```python
from build123d import *

# Parameters (mm, degrees)
SKETCH_1_R           = 2
EXTRUDE_1_DEPTH      = 3
SKETCH_2_R           = 2
EXTRUDE_2_DEPTH      = 3
EXTRUDE_3_DEPTH      = 5
EXTRUDE_3_DEPTH_BACK = 5
SKETCH_4_R           = 2
CUT_EXTRUDE_1_DEPTH  = 31.046838436


with BuildPart() as part:
    # Sketch 1 → Extrude 1 (new body)
    with BuildSketch(Plane(origin=(0, 0, 0), x_dir=(1, 0, 0), z_dir=(0, 1, 0))):
        with BuildLine():
            Line((-11.75, 5.5), (11.75, 5.5))
            ThreePointArc((11.75, 5.5), (16.808303364, 2.159529364), (15.72220169, -3.804157427))
            Line((15.72220169, -3.804157427), (5, -15))
            Line((5, -15), (-5, -15))
            Line((-5, -15), (-15.72220169, -3.804157427))
            ThreePointArc((-15.72220169, -3.804157427), (-16.808303364, 2.159529364), (-11.75, 5.5))
        make_face()
        with Locations(Location((-11.75, 0, 0), (0, 0, 270))):
            Circle(SKETCH_1_R, mode=Mode.SUBTRACT)
        with Locations(Location((11.75, 0, 0), (0, 0, 270))):
            Circle(SKETCH_1_R, mode=Mode.SUBTRACT)
    extrude(amount=EXTRUDE_1_DEPTH)

    # Sketch 2 → Extrude 2 (add)
    with BuildSketch(Plane.XY.offset(15)):
        with BuildLine():
            Line((11.75, 22.5), (-11.75, 22.5))
            ThreePointArc((-11.75, 22.5), (-16.717422464, 19.361083239), (-16.014908335, 13.527168749))
            Line((-16.014908335, 13.527168749), (-5, 0))
            Line((-5, 0), (5, 0))
            Line((5, 0), (16.014908335, 13.527168749))
            ThreePointArc((16.014908335, 13.527168749), (16.717422464, 19.361083239), (11.75, 22.5))
        make_face()
        with Locations((11.75, 17)):
            Circle(SKETCH_2_R, mode=Mode.SUBTRACT)
        with Locations((-11.75, 17)):
            Circle(SKETCH_2_R, mode=Mode.SUBTRACT)
    extrude(amount=-EXTRUDE_2_DEPTH)

    # Sketch 3 → Extrude 3 (add, two sides: drawn at the far end of the back side and taken through both)
    with BuildSketch(Plane(origin=(0, 0, 0), x_dir=(0, 0, -1), z_dir=(1, 0, 0)).offset(-EXTRUDE_3_DEPTH_BACK)):
        Polygon((-12, 13.527168749), (-3.804157427, 3), (-12, 3), align=None)
    extrude(amount=EXTRUDE_3_DEPTH + EXTRUDE_3_DEPTH_BACK)

    # Sketch 4 → Cut-Extrude 1 (cut, through all)
    with BuildSketch(Plane(origin=(0, 3, 0), x_dir=(1, 0, 0), z_dir=(0, 1, 0))):
        with Locations(Location((0, -7.947430558, 0), (0, 0, 90))):
            Circle(SKETCH_4_R)
    extrude(amount=CUT_EXTRUDE_1_DEPTH, mode=Mode.SUBTRACT)


solid = part.part
```
Could you check a few things on this model? Use its own coordinates, in mm. A direction names the side the tool comes from. Round coordinates to 2 decimals unless told otherwise and drop trailing zeros. Write each loop counter-clockwise with the first axis right and the second up, starting at its lowest first coordinate (ties: lowest second). Pieces come first, ordered by that corner, then holes. Notation, with made-up numbers: M 35.25,70.5 L 92.25,70.5 A21 ccw 92.25,100.5 Z; hole C 51.25,74 d3. An arc over 180 degrees is marked long. Answer in a Markdown table with one row per item. Add a question column.
Q1. If I drill on line 1 (X direction, y = 2.25, z = 0); line 2 (Z direction, x = 11, y = 8); line 3 (Y direction, x = 11, z = 7.5), over which ranges is the centre line in solid material (lowest first)? Write a range as from..to.
Q2. Imagine slicing it at D-D (x = -10.5). Please give me the cut outline in (y, z), then the cut area to 3 significant figures.
Q3. If we mould it in two halves opening along Y, with no side actions, what happens to faces 1 (the cylindrical face through (-16.84, 1.48, -2.08)), 2 (the flat face through (0, 3, 8)), 3 (the cylindrical face through (11.49, 18.983, 13.521)), 4 (the cylindrical face through (16.754, 19.282, 13.521))? For each: +Y half, -Y half, draft (parallel to the pull), parting line (faces both ways), or undercut.
Q4. Will these pins go through, and if not, where does the flat tip stop? pin 1 Ø5 at (x, y) = (-11.75, 17) entering from -Z; pin 2 Ø2.5 at (x, z) = (11.75, 0) entering from -Y; pin 3 Ø2 at (x, z) = (0, 8.5) entering from +Y; pin 4 Ø9 at (y, z) = (6.5, 10) entering from -X.
Q5. On a 3-axis mill with a long thin cutter (end or side, diameter ignored), from which of +Z, -Z, +X, -X, +Y, -Y can I reach the whole of each face in a straight line? I mean faces 5 (the flat face through (0, 15, 12)), 6 (the flat face through (10.44, 1.48, 9.32)), 7 (the flat face through (5, 6, 10)). Say none if no direction works.
Q6. Imagine slicing it at B-B (z = 0.75). Please give me the cut outline in (x, y), then the cut area to 3 significant figures.
Q7. Imagine slicing it at C-C (y = 4.75). Please give me the cut outline in (x, z), then the cut area to 3 significant figures.
Q8. Imagine slicing it at A-A (x = 3). Please give me the cut outline in (y, z), then the cut area to 3 significant figures.
Values:
| question | item | result |
|---|---|---|
| 1 | line 1 | -17.25..-13.75, -9.75..9.75, 13.75..17.25 |
| 1 | line 2 | 12..15 |
| 1 | line 3 | 0..3 |
| 2 | outline | M 0,-5.5 L 3,-5.5 L 3,-1.56 L 0,-1.56 Z; M 0,1.56 L 3,1.56 L 3,9.26 L 0,9.26 Z; M 6.75,12 L 15.44,12 L 15.44,15 L 6.75,15 Z; M 18.56,12 L 22.5,12 L 22.5,15 L 18.56,15 Z |
| 2 | area | 72.8 mm^2 |
| 3 | face 1 | draft |
| 3 | face 2 | +Y half |
| 3 | face 3 | undercut |
| 3 | face 4 | parting line |
| 4 | pin 1 | z = 12 |
| 4 | pin 2 | through |
| 4 | pin 3 | y = 3 |
| 4 | pin 4 | x = -13.58 |
| 5 | face 5 | -Z, +Y |
| 5 | face 6 | +Z, +X, -Y |
| 5 | face 7 | -Z, +X, +Y |
| 6 | outline | M -17.2,0 L -13.6,0 L -13.6,3 L -17.2,3 Z; M -9.9,0 L 9.9,0 L 9.9,3 L -9.9,3 Z; M 13.6,0 L 17.2,0 L 17.2,3 L 13.6,3 Z |
| 6 | area | 80.9 mm^2 |
| 7 | outline | M -8.87,12 L -5,12 L -5,5.17 L 5,5.17 L 5,12 L 8.87,12 L 8.87,15 L -8.87,15 Z; hole C 0,7.95 d4 |
| 7 | area | 109 mm^2 |
| 8 | outline | M 0,-5.5 L 3,-5.5 L 3,3.8 L 13.53,12 L 22.5,12 L 22.5,15 L 0,15 Z |
| 8 | area | 163 mm^2 |
